Print and shaded views of the part. All mm, measured from the part's lowest x, y and z. A direction names the side the tool comes from. Coordinates: 2 decimals unless noted, no trailing zeros. Write each loop counter-clockwise with the first axis right and the second up, starting at its lowest first coordinate (ties: lowest second). Pieces come first, ordered by that corner, then holes. Notation, with made-up numbers: (18, 36) -> (33, 36) arc R25 cw to (33, 61) -> close; hole circle Ø9 at (45, -19). An arc over 180 degrees is marked (long way). Write item = value, one per line.
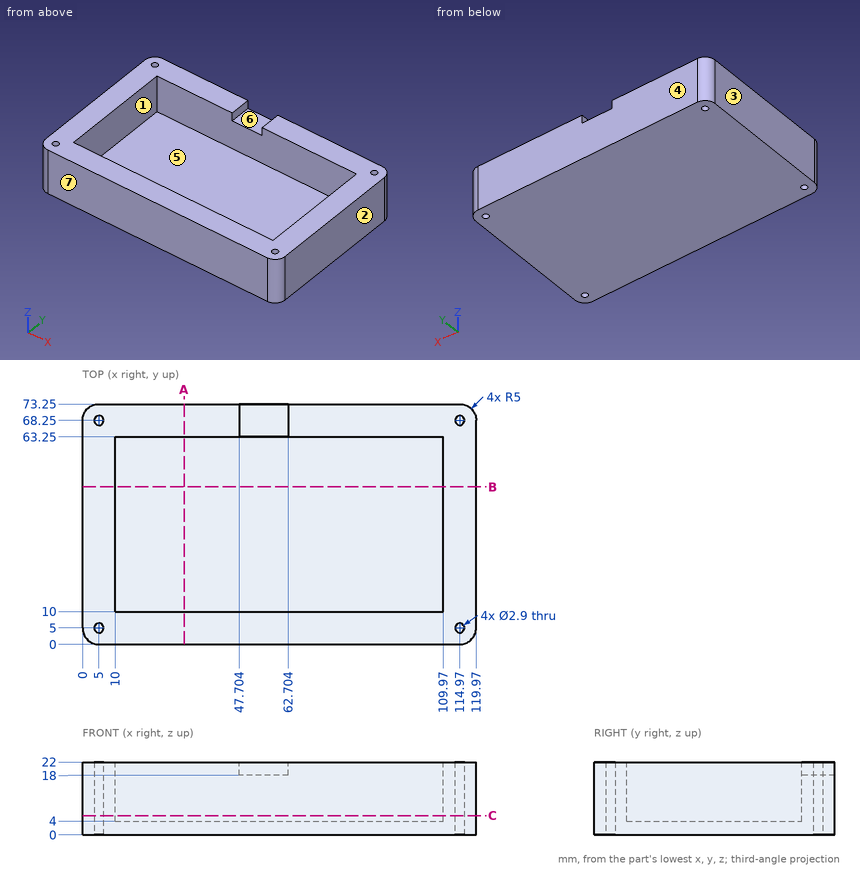
Q1. Mould opens along X. For the marked faces 1, 2, 3 and 4 say: released by +X, released by -X, zero draft, split by the parting line, or undercut.
Model answer:
face_1 = undercut
face_2 = released by +X
face_3 = released by -X
face_4 = zero draft
Q2. Probe line 1 (Y direction, x = 114.97, z = 6.75); line 2 (X direction, y = 68.25, z = 12.5); line 3 (X direction, y = 56, z = 4.75). List the from-to ranges inside material, lowest first. Write a range as from..to.
Model answer:
line_1 = 0..3.55, 6.45..66.8, 69.7..73.25
line_2 = 0..3.55, 6.45..113.52, 116.42..119.97
line_3 = 0..10, 109.97..119.97
Q3. Which spindle directions (+Z, -Z, +X, -X, +Y, -Y) get a long thin tool onto all of the face, cutting with end or side? Do the marked faces 5, 6 and 7. Say none if no direction does.
Model answer:
face_5 = +Z
face_6 = +Z, +Y
face_7 = +Z, -Z, +X, -X, -Y
Q4. Saw through at C-C on z = 5.75. Give the cut face in (x, y), and give its area (3 significant figures).
Model answer:
outline = (0, 5) arc R5 ccw to (5, 0) -> (114.97, 0) arc R5 ccw to (119.97, 5) -> (119.97, 68.25) arc R5 ccw to (114.97, 73.25) -> (5, 73.25) arc R5 ccw to (0, 68.25) -> close; hole circle Ø2.9 at (5, 5); hole circle Ø2.9 at (5, 68.25); hole (10, 10) -> (109.97, 10) -> (109.97, 63.25) -> (10, 63.25) -> close; hole circle Ø2.9 at (114.97, 5); hole circle Ø2.9 at (114.97, 68.25)
area = 3,420 mm²
Q5. Saw through at A-A on x = 31. Give the cut face in (y, z), and give its area (3 significant figures).
Model answer:
outline = (0, 0) -> (73.25, 0) -> (73.25, 22) -> (63.25, 22) -> (63.25, 4) -> (10, 4) -> (10, 22) -> (0, 22) -> close
area = 653 mm²
Q6. Pin check, flat tips, straight feed: pin 1 (2 mm diameter, centred on y = 70, z = 20, fed in from -X); pin 2 (1.7 mm diameter, centred on x = 5, y = 68.25, fed in from +Z); pin 3 (16 mm diameter, centred on x = 69.5, y = 43.5, fed in from +Z); pin 4 (5 mm diameter, centred on x = 53.5, y = 66, fed in from +Z). Stop position of each tip, or through.
Model answer:
pin_1 = 0.06
pin_2 = through
pin_3 = 4
pin_4 = 18
Q7. Saw through at B-B on y = 48. Give the cut face in (x, z).
Model answer:
outline = (0, 0) -> (119.97, 0) -> (119.97, 22) -> (109.97, 22) -> (109.97, 4) -> (10, 4) -> (10, 22) -> (0, 22) -> close
